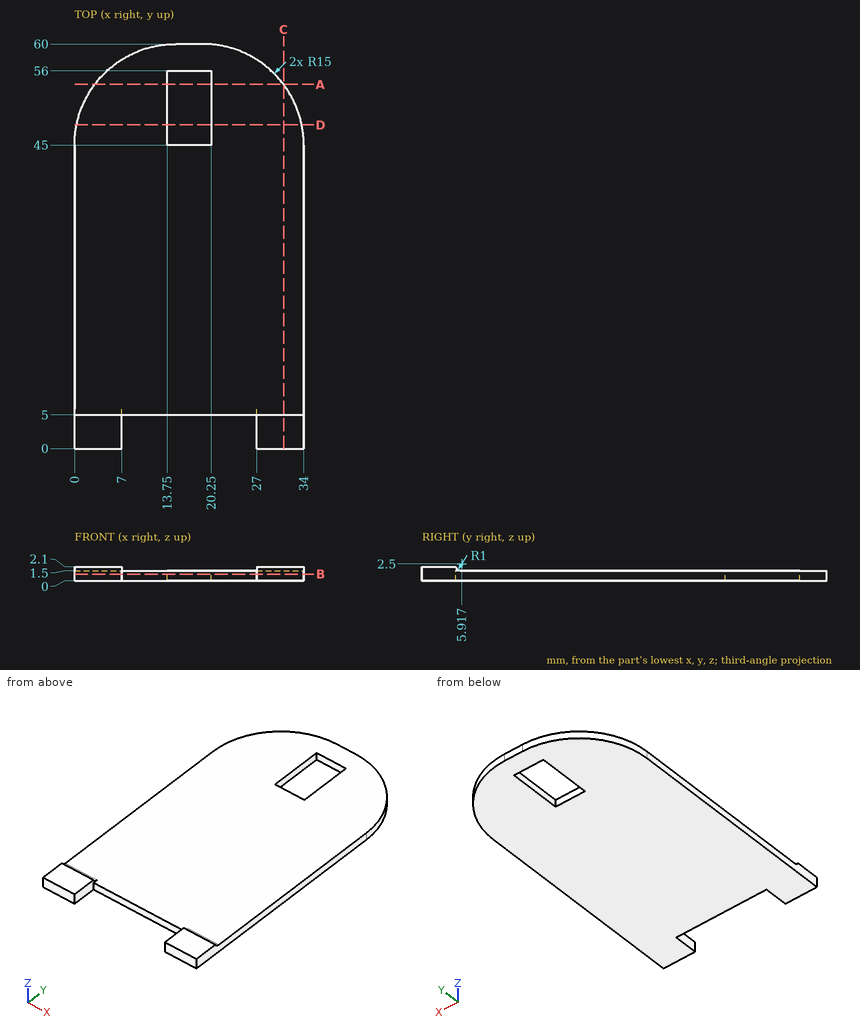
Input: dimensioned drawing with shaded views. Units: mm. Origin: part minimum x, y, z. Give positions to 0.01 mm unless a question says otherwise; leave off trailing zeros. Write each loop counter-clockwise with the first axis right and the second up, starting at its lowest first coordinate (ties: lowest second). Pieces come first, ordered by that corner, then holes. Notation, with made-up numbers: (5.25, 81) -> (53.25, 81) arc R16 cw to (53.25, 97) -> close; hole circle Ø3 at (46.25, 78.25). An arc over 180 degrees is marked (long way). Answer as a JSON object with one key per item and string values.
1. Cut plane C-C on x = 31. Output: boundary loops of the cut face in (y, z).
Ans:
{"outline": "(0, 0) -> (54, 0) -> (54, 1.5) -> (5.92, 1.5) arc R1 cw to (5, 2.1) -> (0, 2.1) -> close"}
2. Contact query for flat-ended pins moving along their axis: pin 1 (1.2 mm diameter, centred on x = 14, z = 0.5, fed in from -Y); pin 2 (0.8 mm diameter, centred on y = 52.5, z = 1, fed in from -X); pin 3 (1 mm diameter, centred on x = 26.5, z = 1.5, fed in from +Y). Output: stop coordinate, or through.
Ans:
{"pin 1": "stops at y = 5", "pin 2": "stops at x = 1.79", "pin 3": "stops at y = 58.27"}
3. Cut plane A-A on y = 54. Output: boundary loops of the cut face in (x, z).
Ans:
{"outline": "(3, 0) -> (13.75, 0) -> (13.75, 1.5) -> (3, 1.5) -> close; (20.25, 0) -> (31, 0) -> (31, 1.5) -> (20.25, 1.5) -> close"}
4. Cut plane B-B on z = 1. Output: boundary loops of the cut face in (x, y), and give its area (3 significant figures).
Ans:
{"outline": "(0, 0) -> (7, 0) -> (7, 5) -> (27, 5) -> (27, 0) -> (34, 0) -> (34, 45) arc R15 ccw to (19, 60) -> (15, 60) arc R15 ccw to (0, 45) -> close; hole (13.75, 45) -> (20.25, 45) -> (20.25, 56) -> (13.75, 56) -> close", "area": "1,770 mm^2"}
5. Cut plane D-D on y = 48. Output: boundary loops of the cut face in (x, z).
Ans:
{"outline": "(0.3, 0) -> (13.75, 0) -> (13.75, 1.5) -> (0.3, 1.5) -> close; (20.25, 0) -> (33.7, 0) -> (33.7, 1.5) -> (20.25, 1.5) -> close"}
6. Ray query, probe 1 along Y at (x, z) = (15, 1.15); probe 2 along Z at (x, y) = (13, 11); probe 3 along Y at (x, z) = (23, 0.2). Return the intervals inside material, ascending. Write a range as from..to.
Ans:
{"probe 1": "y = 5..45, 56..60", "probe 2": "z = 0..1.5", "probe 3": "y = 5..59.46"}
